Can you work these out from the drawing? Everything is in mm from the part's minimum corner. Round coordinates to 2 decimals unless told otherwise and drop trailing zeros. Write each loop counter-clockwise with the first axis right and the second up, starting at its lowest first coordinate (ties: lowest second). Pieces come first, ordered by that corner, then holes. Notation, with made-up numbers: (-14, 34.5) -> (29, 34.5) arc R24 cw to (29, 46.5) -> close; hole circle Ø4 at (36.5, 1.5). An arc over 180 degrees is marked (long way). Answer as CSV lines item,"result". Start each with the question number.
Q1. Imagine slicing it at A-A on z = 6. Please give me the cut outline in (x, y), and give its area (3 significant figures).
Q2. Imagine slicing it at B-B on x = 152. Please give me the cut outline in (y, z) (3 decimals).
Q3. If I drill on line 1 (Y direction, x = 163.5, z = 0.5); line 2 (Y direction, x = 336, z = 4.5), over which ranges is the centre line in solid material (lowest first)? Write a range as [from, to].
Q4. Will these pins go through, and if not, where does the flat tip stop? pin 1 Ø3 at (x, z) = (195, 5.5) entering from -Y; pin 2 Ø5 at (y, z) = (337.5, 5.5) entering from +X.
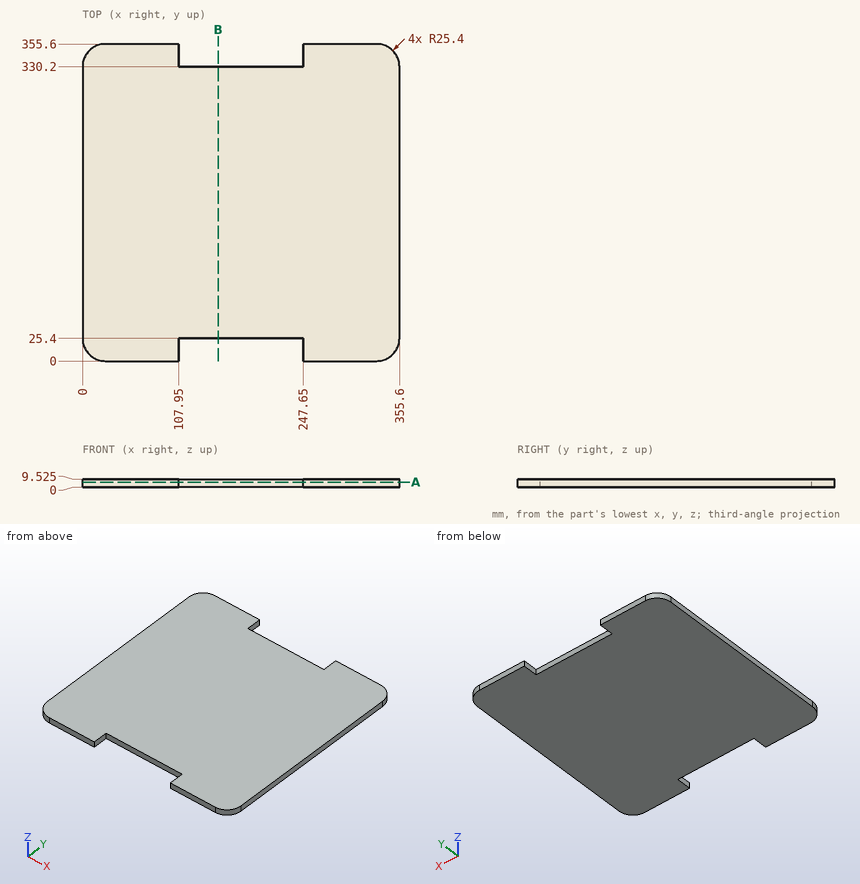
Checks:
1,outline,"(0, 25.4) arc R25.4 ccw to (25.4, 0) -> (107.95, 0) -> (107.95, 25.4) -> (247.65, 25.4) -> (247.65, 0) -> (330.2, 0) arc R25.4 ccw to (355.6, 25.4) -> (355.6, 330.2) arc R25.4 ccw to (330.2, 355.6) -> (247.65, 355.6) -> (247.65, 330.2) -> (107.95, 330.2) -> (107.95, 355.6) -> (25.4, 355.6) arc R25.4 ccw to (0, 330.2) -> close"
1,area,"119,000 mm^2"
2,outline,"(25.4, 0) -> (330.2, 0) -> (330.2, 9.525) -> (25.4, 9.525) -> close"
3,line 1,"[25.4, 330.2]"
3,line 2,"[0.67, 354.93]"
4,pin 1,"y = 25.4"
4,pin 2,"x = 355.14"
